Design review of the part built by this model. Coordinates are the model's own, in mm. A direction names the side the tool comes from. Coordinates: 2 decimals unless noted, no trailing zeros. Order: outer loops, then holes, each group sorted by start corner. A loop starts at its lowest first (then second) coordinate and runs counter-clockwise, first axis right, second up. Notation, with made-up numbers: (32.25, 56) -> (47.25, 56) arc R26 ccw to (47.25, 91) -> close; hole circle Ø11 at (75.25, 59). An arc over 180 degrees is marked (long way). Write item = value, one per line.
Autodesk Inventor part; units mm, degrees
ref_plane "YZ Plane" through (0, 0, 0) normal (1, 0, 0) x (0, 1, 0)
ref_plane "XZ Plane" through (0, 0, 0) normal (0, 1, 0) x (-1, 0, 0)
ref_plane "XY Plane" through (0, 0, 0) normal (0, 0, 1) x (1, 0, 0)
sketch "Sketch1" plane through (0, 0, 0) normal (0, 0, 1) x (1, 0, 0)
  line L0 (24.13, -26.67) -> (-24.13, -26.67)
  line L1 (-24.13, -26.67) -> (-24.13, 26.67)
  line L2 (-24.13, 26.67) -> (24.13, 26.67)
  line L3 (24.13, 26.67) -> (24.13, -26.67)
  line L4 (0, 37.338) -> (0, -37.338)
  line L5 (-33.782, 0) -> (33.782, 0)
  dimension "d0" = 53.34
  dimension "d1" = 48.26
extrude "Extrusion1" add sketch "Sketch1" against normal blind 66.675
shell "Shell1" thickness 1.905 removed faces 1 at (-8.0433, 8.89, -66.675)
sketch "Sketch2" plane through (0, 0, 0) normal (0, 0, 1) x (1, 0, 0)
  point P0 (0, 0)
  point P1 (0, 0)
hole "Hole1" at (0, 0, 0) direction (0, 0, -1) diameter 44.45 end through all
sketch "Sketch3" plane through (24.13, -26.67, 0) normal (1, 0, 0) x (0, 0, -1)
  line L0 (0, 0) -> (66.675, 0)
  line L1 (50.8, 0) -> (50.8, 10.16)
  line L2 (50.8, 10.16) -> (66.675, 10.16)
  line L3 (66.675, 1.905) -> (66.675, 51.435)
  line L4 (0, 53.34) -> (66.675, 53.34)
  line L5 (50.8, 53.34) -> (50.8, 46.99)
  line L6 (50.8, 46.99) -> (66.675, 46.99)
  line L7 (66.675, 53.34) -> (66.675, 0)
  point P0 (0, 26.67)
  dimension "d12" = 10.16
  dimension "d13" = 6.35
  dimension "d14" = 15.875
extrude "Extrusion2" cut sketch "Sketch3" against normal up to next
properties part number "EStop Mount" material "PBT Plastic"
(1) The part is to be moulded in two halves that separate along X. For faces 1 (the flat face through (2, 23, -1.905)), 2 (the flat face through (-2, 25, -50.8)), 3 (the flat face through (-24.13, 0, -33)), say which applies: released by +X, released by -X, zero draft, split by the parting line, or undercut.
Report:
face_1 = undercut
face_2 = zero draft
face_3 = released by -X
(2) Insertion check: pin 1 (1 mm diameter, centred on x = -23, z = -59, fed in from +Y); pin 2 (0.6 mm diameter, centred on x = 23.5, z = -61.5, fed in from -Y); pin 3 (3 mm diameter, centred on x = -4.5, y = 22, fed in from -Z) (3 decimals). Each pin has a flat end and moves straight along its axis. Give the tip position at first contact, or say it passes through.
Report:
pin_1 = 20.32
pin_2 = -16.51
pin_3 = -1.905
(3) We need section B-B (z = -39). Write out the cut boundary in (x, y) (3 decimals).
Report:
outline = (-24.13, -26.67) -> (24.13, -26.67) -> (24.13, 26.67) -> (-24.13, 26.67) -> close; hole (-22.225, -24.765) -> (22.225, -24.765) -> (22.225, 24.765) -> (-22.225, 24.765) -> close
(4) We need section C-C (y = 14.5). Write out the cut boundary in (x, z) (3 decimals).
Report:
outline = (-24.13, -66.675) -> (-22.225, -66.675) -> (-22.225, -1.905) -> (-16.843, -1.905) -> (-16.843, 0) -> (-24.13, 0) -> close; (16.843, -1.905) -> (22.225, -1.905) -> (22.225, -66.675) -> (24.13, -66.675) -> (24.13, 0) -> (16.843, 0) -> close
(5) For L1, parallel to Y at x = 13, z = -36 (3 decimals); L2, parallel to Y at x = 0, z = -1 (3 decimals); L3, parallel to X at y = 11.5, z = -24.5 (3 decimals), list the stretches that pass through material, from the lowest coordinate up.
Report:
L1 = -26.67 to -24.765, 24.765 to 26.67
L2 = -26.67 to -22.225, 22.225 to 26.67
L3 = -24.13 to -22.225, 22.225 to 24.13
(6) For faces 4 (the flat face through (23, -16.51, -59)), 5 (the flat face through (24.13, 0, -33)), 6 (the flat face through (0, 24.765, -26)), list the 3-axis set-ups (+Z, -Z, +X, -X, +Y, -Y) from which the entire face can be reached by the end or side of a thin tool; tool diameter is ignored.
Report:
face_4 = -Z, +X, -X, -Y
face_5 = +Z, -Z, +X, +Y, -Y
face_6 = -Z
(7) We need section A-A (x = 0). Write out the cut boundary in (y, z) (3 decimals), and give its area (3 significant figures).
Report:
outline = (-26.67, -50.8) -> (-24.765, -50.8) -> (-24.765, -1.905) -> (-22.225, -1.905) -> (-22.225, 0) -> (-26.67, 0) -> close; (22.225, -1.905) -> (24.765, -1.905) -> (24.765, -50.8) -> (26.67, -50.8) -> (26.67, 0) -> (22.225, 0) -> close
area = 203 mm²
